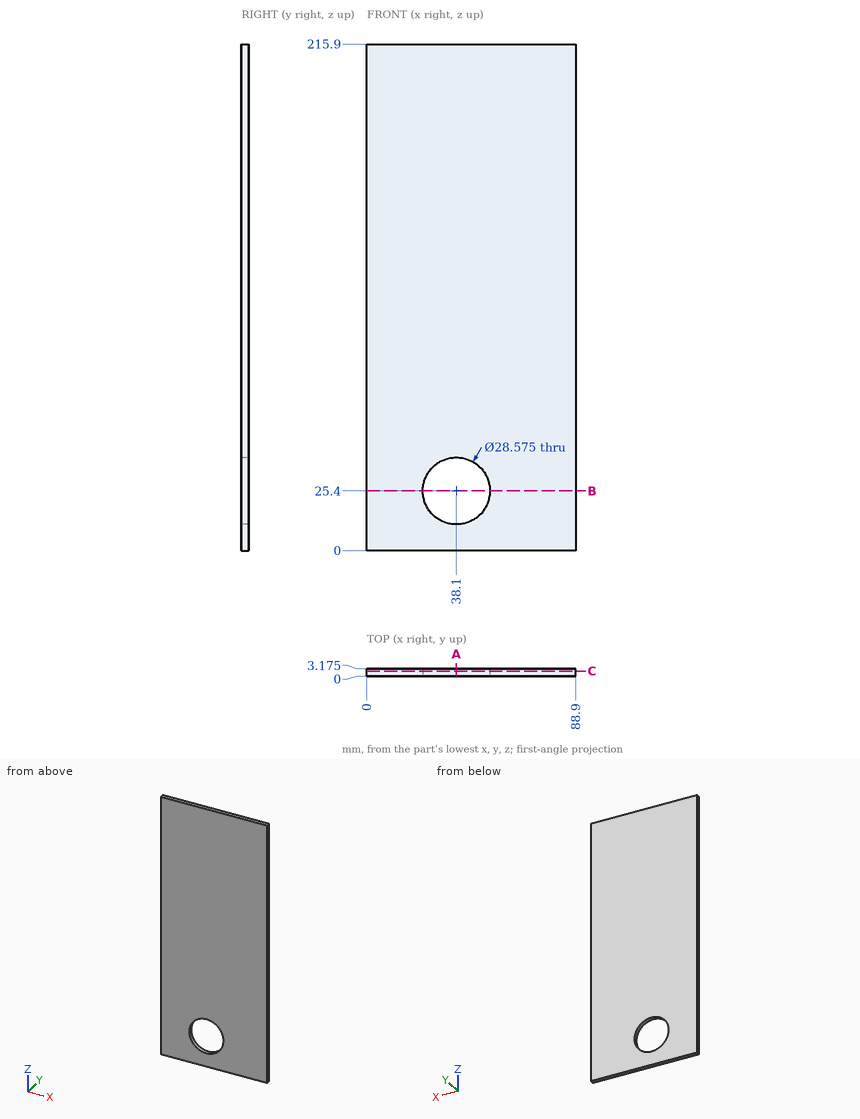
For this review, use the dimensioned drawing (mm, ordinates from the lowest corner) and the shaded views. Round coordinates to 2 decimals unless told otherwise and drop trailing zeros. Order: outer loops, then holes, each group sorted by start corner. A loop starts at its lowest first (then second) coordinate and runs counter-clockwise, first axis right, second up. Notation, with made-up numbers: M 68,60.25 L 120,60.25 A24 ccw 120,70.25 Z; hole C 70.5,3.5 d7. An arc over 180 degrees is marked long. Use a Markdown table: item, result. Add a question column.
Item 1: To check wall thickness, follow line 1 along X through (y, z) = (1.2, 25.4); line 2 along Z through (x, y) = (47.5, 2.65); line 3 along X through (y, z) = (1.15, 17). State the ranges of each line that lie inside material, in increasing order.
Item 2: Add section A-A, the plane x = 38.1. Give the boundary of the cut face in (y, z) (1 decimal), then the cut area to 3 significant figures.
Item 3: Add section C-C, the plane y = 2.1. Give the boundary of the cut face in (x, z) (1 decimal).
Item 4: Add section B-B, the plane z = 25.4. Give the boundary of the cut face in (x, y) (1 decimal).
Geometry results:
| question | item | result |
|---|---|---|
| 1 | line 1 | x = 0 to 23.81, 52.39 to 88.9 |
| 1 | line 2 | z = 0 to 14.64, 36.16 to 215.9 |
| 1 | line 3 | x = 0 to 26.54, 49.66 to 88.9 |
| 2 | outline | M 0,0 L 3.2,0 L 3.2,11.1 L 0,11.1 Z; M 0,39.7 L 3.2,39.7 L 3.2,215.9 L 0,215.9 Z |
| 2 | area | 595 mm² |
| 3 | outline | M 0,0 L 88.9,0 L 88.9,215.9 L 0,215.9 Z; hole C 38.1,25.4 d28.6 |
| 4 | outline | M 0,0 L 23.8,0 L 23.8,3.2 L 0,3.2 Z; M 52.4,0 L 88.9,0 L 88.9,3.2 L 52.4,3.2 Z |
